from build123d import *

# Parameters (mm, degrees)
F0_R         = 7.62
F1_DEPTH     = 19.05
F3_DEPTH     = 12.7
F4_SIZE      = 1.27
F5_T1_DEPTH  = 8.5497045256
F5_T3_DEPTH  = 8.5497045256
F5_T5_DEPTH  = 8.5497045256
F5_T7_DEPTH  = 8.5497045256
F5_T12_DEPTH = 8.5497045256
F5_S13_R     = 7.62
F5_T14_DEPTH = 6
F5_T18_DEPTH = 8.5497045256
F5_S19_R     = 7.62
F5_T20_DEPTH = 6
F5_T24_DEPTH = 8.5497045256
F5_S25_R     = 7.62
F5_T26_DEPTH = 6
F5_T30_DEPTH = 8.5497045256
F5_S31_R     = 7.62
F5_T32_DEPTH = 6
F5_T36_DEPTH = 8.5497045256
F5_S37_R     = 7.62
F5_T38_DEPTH = 6
F5_T42_DEPTH = 8.5497045256
F5_S43_R     = 7.62
F5_T44_DEPTH = 6
F6_R         = 7.62
F7_DEPTH     = 12.7
F8_R         = 6.35
F9_DEPTH     = 44.4510001


# Not quite as in the source:
# - a fillet or chamfer that OpenCascade refuses, or shapes differently, is made with other operations: its cross-section is extruded or revolved along the edge and cut away or added


with BuildPart() as f1:
    # F0 (on Front) → F1 (new body)
    with BuildSketch(Plane.XZ):
        Circle(F0_R)
    extrude(amount=F1_DEPTH)

    # F2 (on face) → F3 (join)
    with BuildSketch(Plane.XZ.offset(19.05)):
        with BuildLine():
            Line((7.8629215405, 3.9488814679), (4.1872753391, 6.3664059904))
            ThreePointArc((4.1872753391, 6.3664059904), (6.7071394083, 3.6164459015), (7.62, 0))
            ThreePointArc((7.62, 0), (7.616776064, -0.2216357159), (7.6071069841, -0.4430838887))
            Line((7.6071069841, -0.4430838887), (7.8629215405, 3.9488814679))
        make_face()
        with BuildLine():
            ThreePointArc((4.1872753391, 6.3664059904), (0.4430838236, 7.6071069879), (-3.4198316443, 6.8094898138))
            ThreePointArc((-3.4198316443, 6.8094898138), (-6.3664059346, 4.187275424), (-7.6071069765, 0.4430840189))
            ThreePointArc((-7.6071069765, 0.4430840189), (-6.8094898664, -3.4198315396), (-4.187275378, -6.3664059648))
            ThreePointArc((-4.187275378, -6.3664059648), (-0.4430838337, -7.6071069873), (3.419831668, -6.8094898019))
            ThreePointArc((3.419831668, -6.8094898019), (6.3664059777, -4.1872753585), (7.6071069841, -0.4430838887))
            ThreePointArc((7.6071069841, -0.4430838887), (7.616776064, -0.2216357159), (7.62, 0))
            ThreePointArc((7.62, 0), (6.7071394083, 3.6164459015), (4.1872753391, 6.3664059904))
        make_face()
        with BuildLine():
            ThreePointArc((7.6071069841, -0.4430838887), (6.3664059777, -4.1872753585), (3.419831668, -6.8094898019))
            Line((3.419831668, -6.8094898019), (7.351292438, -4.8350490681))
            Line((7.351292438, -4.8350490681), (7.6071069841, -0.4430838887))
        make_face()
        with BuildLine():
            ThreePointArc((3.419831668, -6.8094898019), (-0.4430838337, -7.6071069873), (-4.187275378, -6.3664059648))
            Line((-4.187275378, -6.3664059648), (-0.5116291025, -8.783930536))
            Line((-0.5116291025, -8.783930536), (3.419831668, -6.8094898019))
        make_face()
        with BuildLine():
            ThreePointArc((-4.187275378, -6.3664059648), (-6.8094898664, -3.4198315396), (-7.6071069765, 0.4430840189))
            Line((-7.6071069765, 0.4430840189), (-7.8629215405, -3.9488814679))
            Line((-7.8629215405, -3.9488814679), (-4.187275378, -6.3664059648))
        make_face()
        with BuildLine():
            Line((-3.4198316443, 6.8094898138), (-7.351292438, 4.8350490681))
            Line((-7.351292438, 4.8350490681), (-7.6071069765, 0.4430840189))
            ThreePointArc((-7.6071069765, 0.4430840189), (-6.3664059346, 4.187275424), (-3.4198316443, 6.8094898138))
        make_face()
        with BuildLine():
            Line((0.5116291025, 8.783930536), (-3.4198316443, 6.8094898138))
            ThreePointArc((-3.4198316443, 6.8094898138), (0.4430838236, 7.6071069879), (4.1872753391, 6.3664059904))
            Line((4.1872753391, 6.3664059904), (0.5116291025, 8.783930536))
        make_face()
    extrude(amount=F3_DEPTH)

    # F4
    f4_edges = [f1.edges().sort_by_distance(p)[0] for p in [
        (7.862922, -25.4, 3.948881),
        (7.351292, -25.4, -4.835049),
        (-0.511629, -25.4, -8.783931),
        (-7.862922, -25.4, -3.948881),
        (-7.351292, -25.4, 4.835049),
        (0.511629, -25.4, 8.783931),
    ]]
    chamfer(f4_edges, length=F4_SIZE)

    # F5: fillet of radius 1.27 on 12 edges, made by hand

    # F5_s2 → F5_t1 (cut)
    with BuildSketch(Plane(origin=(1.918540045, 0, -3.8201526101), x_dir=(0, 1, 0), z_dir=(-0.4487968068, 0, 0.8936338323))):
        with BuildLine():
            ThreePointArc((-30.48, -8.1638181024), (-31.3780256121, -7.7918437146), (-31.75, -6.8938181024))
            Line((-31.75, -6.8938181024), (-31.75, -8.1638181024))
            Line((-31.75, -8.1638181024), (-30.48, -8.1638181024))
        make_face()
        with BuildLine():
            ThreePointArc((-31.75, 6.8938181024), (-31.3780256121, 7.7918437146), (-30.48, 8.1638181024))
            Line((-30.48, 8.1638181024), (-31.75, 8.1638181024))
            Line((-31.75, 8.1638181024), (-31.75, 6.8938181024))
        make_face()
    extrude(amount=F5_T1_DEPTH, mode=Mode.SUBTRACT)

    # F5_s4 → F5_t3 (cut)
    with BuildSketch(Plane(origin=(4.2676192292, 0, -0.2485718879), x_dir=(0, 1, 0), z_dir=(-0.9983080038, 0, 0.0581474803))):
        with BuildLine():
            ThreePointArc((-31.75, -6.8938181024), (-31.3780256121, -7.7918437146), (-30.48, -8.1638181024))
            Line((-30.48, -8.1638181024), (-31.75, -8.1638181024))
            Line((-31.75, -8.1638181024), (-31.75, -6.8938181024))
        make_face()
        with BuildLine():
            ThreePointArc((-31.75, 6.8938181024), (-31.3780256121, 7.7918437146), (-30.48, 8.1638181024))
            Line((-30.48, 8.1638181024), (-31.75, 8.1638181024))
            Line((-31.75, 8.1638181024), (-31.75, 6.8938181024))
        make_face()
    extrude(amount=F5_T3_DEPTH, mode=Mode.SUBTRACT)

    # F5_s6 → F5_t5 (cut)
    with BuildSketch(Plane(origin=(-2.3490791841, 0, -3.5715807222), x_dir=(0, 1, 0), z_dir=(0.5495111971, 0, 0.835486352))):
        with BuildLine():
            ThreePointArc((-31.75, 6.8938181024), (-31.3780256121, 7.7918437146), (-30.48, 8.1638181024))
            Line((-30.48, 8.1638181024), (-31.75, 8.1638181024))
            Line((-31.75, 8.1638181024), (-31.75, 6.8938181024))
        make_face()
    extrude(amount=F5_T5_DEPTH, mode=Mode.SUBTRACT)

    # F5_s8 → F5_t7 (cut)
    with BuildSketch(Plane(origin=(2.3490791841, 0, 3.5715807222), x_dir=(0, 1, 0), z_dir=(-0.5495111971, 0, -0.835486352))):
        with BuildLine():
            ThreePointArc((-30.48, 8.1638181024), (-31.3780256121, 7.7918437146), (-31.75, 6.8938181024))
            Line((-31.75, 6.8938181024), (-31.75, 8.1638181024))
            Line((-31.75, 8.1638181024), (-30.48, 8.1638181024))
        make_face()
    extrude(amount=F5_T7_DEPTH, mode=Mode.SUBTRACT)


with BuildPart() as f5_tool10:
    # F5_s11 → F5_t12 (new body)
    with BuildSketch(Plane(origin=(4.2676192292, 0, -0.2485718879), x_dir=(0, 1, 0), z_dir=(-0.9983080038, 0, 0.0581474803))):
        with BuildLine():
            ThreePointArc((-19.05, -6.8938181024), (-19.4219743879, -7.7918437146), (-20.32, -8.1638181024))
            Line((-20.32, -8.1638181024), (-19.05, -8.1638181024))
            Line((-19.05, -8.1638181024), (-19.05, -6.8938181024))
        make_face()
    extrude(amount=F5_T12_DEPTH)

    # F5_s13 → F5_t14 (cut, symmetric)
    with BuildSketch(Plane.XZ.offset(19.7)):
        Circle(F5_S13_R)
    extrude(amount=F5_T14_DEPTH, both=True, mode=Mode.SUBTRACT)


with BuildPart() as f1_1:
    add(f1.part)

    # F5_t9: cut F5_tool10
    add(f5_tool10.part, mode=Mode.SUBTRACT)


with BuildPart() as f5_tool16:
    # F5_s17 → F5_t18 (new body)
    with BuildSketch(Plane(origin=(-2.3490791841, 0, -3.5715807222), x_dir=(0, 1, 0), z_dir=(0.5495111971, 0, 0.835486352))):
        with BuildLine():
            ThreePointArc((-19.05, 6.8938181024), (-19.4219743879, 7.7918437146), (-20.32, 8.1638181024))
            Line((-20.32, 8.1638181024), (-19.05, 8.1638181024))
            Line((-19.05, 8.1638181024), (-19.05, 6.8938181024))
        make_face()
    extrude(amount=F5_T18_DEPTH)

    # F5_s19 → F5_t20 (cut, symmetric)
    with BuildSketch(Plane.XZ.offset(19.7)):
        Circle(F5_S19_R)
    extrude(amount=F5_T20_DEPTH, both=True, mode=Mode.SUBTRACT)


with BuildPart() as f1_2:
    add(f1_1.part)

    # F5_t15: cut F5_tool16
    add(f5_tool16.part, mode=Mode.SUBTRACT)


with BuildPart() as f5_tool22:
    # F5_s23 → F5_t24 (new body)
    with BuildSketch(Plane(origin=(1.918540045, 0, -3.8201526101), x_dir=(0, 1, 0), z_dir=(-0.4487968068, 0, 0.8936338323))):
        with BuildLine():
            ThreePointArc((-19.05, 6.8938181024), (-19.4219743879, 7.7918437146), (-20.32, 8.1638181024))
            Line((-20.32, 8.1638181024), (-19.05, 8.1638181024))
            Line((-19.05, 8.1638181024), (-19.05, 6.8938181024))
        make_face()
    extrude(amount=F5_T24_DEPTH)

    # F5_s25 → F5_t26 (cut, symmetric)
    with BuildSketch(Plane.XZ.offset(19.7)):
        Circle(F5_S25_R)
    extrude(amount=F5_T26_DEPTH, both=True, mode=Mode.SUBTRACT)


with BuildPart() as f1_3:
    add(f1_2.part)

    # F5_t21: cut F5_tool22
    add(f5_tool22.part, mode=Mode.SUBTRACT)


with BuildPart() as f5_tool28:
    # F5_s29 → F5_t30 (new body)
    with BuildSketch(Plane(origin=(4.2676192292, 0, -0.2485718879), x_dir=(0, 1, 0), z_dir=(-0.9983080038, 0, 0.0581474803))):
        with BuildLine():
            ThreePointArc((-19.05, 6.8938181024), (-19.4219743879, 7.7918437146), (-20.32, 8.1638181024))
            Line((-20.32, 8.1638181024), (-19.05, 8.1638181024))
            Line((-19.05, 8.1638181024), (-19.05, 6.8938181024))
        make_face()
    extrude(amount=F5_T30_DEPTH)

    # F5_s31 → F5_t32 (cut, symmetric)
    with BuildSketch(Plane.XZ.offset(19.7)):
        Circle(F5_S31_R)
    extrude(amount=F5_T32_DEPTH, both=True, mode=Mode.SUBTRACT)


with BuildPart() as f1_4:
    add(f1_3.part)

    # F5_t27: cut F5_tool28
    add(f5_tool28.part, mode=Mode.SUBTRACT)


with BuildPart() as f5_tool34:
    # F5_s35 → F5_t36 (new body)
    with BuildSketch(Plane(origin=(2.3490791841, 0, 3.5715807222), x_dir=(0, 1, 0), z_dir=(-0.5495111971, 0, -0.835486352))):
        with BuildLine():
            ThreePointArc((-19.05, 6.8938181024), (-19.4219743879, 7.7918437146), (-20.32, 8.1638181024))
            Line((-20.32, 8.1638181024), (-19.05, 8.1638181024))
            Line((-19.05, 8.1638181024), (-19.05, 6.8938181024))
        make_face()
    extrude(amount=F5_T36_DEPTH)

    # F5_s37 → F5_t38 (cut, symmetric)
    with BuildSketch(Plane.XZ.offset(19.7)):
        Circle(F5_S37_R)
    extrude(amount=F5_T38_DEPTH, both=True, mode=Mode.SUBTRACT)


with BuildPart() as f1_5:
    add(f1_4.part)

    # F5_t33: cut F5_tool34
    add(f5_tool34.part, mode=Mode.SUBTRACT)


with BuildPart() as f5_tool40:
    # F5_s41 → F5_t42 (new body)
    with BuildSketch(Plane(origin=(1.918540045, 0, -3.8201526101), x_dir=(0, 1, 0), z_dir=(-0.4487968068, 0, 0.8936338323))):
        with BuildLine():
            ThreePointArc((-19.05, -6.8938181024), (-19.4219743879, -7.7918437146), (-20.32, -8.1638181024))
            Line((-20.32, -8.1638181024), (-19.05, -8.1638181024))
            Line((-19.05, -8.1638181024), (-19.05, -6.8938181024))
        make_face()
    extrude(amount=F5_T42_DEPTH)

    # F5_s43 → F5_t44 (cut, symmetric)
    with BuildSketch(Plane.XZ.offset(19.7)):
        Circle(F5_S43_R)
    extrude(amount=F5_T44_DEPTH, both=True, mode=Mode.SUBTRACT)


with BuildPart() as f1_6:
    add(f1_5.part)

    # F5_t39: cut F5_tool40
    add(f5_tool40.part, mode=Mode.SUBTRACT)

    # F6 (on face) → F7 (join)
    with BuildSketch(Plane.XZ.offset(31.75)):
        Circle(F6_R)
    extrude(amount=F7_DEPTH)

    # F8 (on face) → F9 (cut, through all)
    with BuildSketch(Plane.XZ.offset(44.45)):
        Circle(F8_R)
    extrude(amount=-F9_DEPTH, mode=Mode.SUBTRACT)


solid = f1_6.part
Geometry: final body of the model. Coordinates: model frame, mm. A direction names the side the tool comes from. Round coordinates to 2 decimals unless told otherwise and drop trailing zeros. Loops run counter-clockwise (first coordinate to the right, second up) from the corner with the lowest first, then second, coordinate; pieces in that order, holes last. Notation, with made-up numbers: M -33,89.25 L -29,89.25 A18 cw -29,96.25 Z; hole C 52,-33 d8. An arc over 180 degrees is marked long. Put each result on its own line as item: value. Start each with the question number.
(1) Draft query along X for faces 4 (the face through (-6.8, -31.5, -3.5)), 5 (the face through (0.46, -25.33, 8.15)), 6 (the face through (-1.65, -38.01, -7.44)). Return one class per face: +X half, -X half, draft (parallel to the pull), parting line (faces both ways), or undercut.
(2) Material intervals for line 1 along Z through (x, y) = (0, -17); line 2 along X through (y, z) = (-1.5, 5), sorted ascending. Write a range as [from, to].
(3) Section query B-B (y = -14). Return loops of the section in (x, z).
(4) Section query A-A (y = -21). Return loops of the section in (x, z), then the cut area to 3 significant figures.
(5) Set-up query: faces 1 (the face through (7.302, -25.329, 3.65)), 2 (the face through (-1.65, -9.5, -7.44)), 3 (the face through (-6.38, -31.53, 4.14)). Return all of +Z, -Z, +X, -X, +Y, -Y with unobstructed straight access to the full face (end or side cutting, diameter ignored); none if empty.
(6) Contact query for flat-ended pins moving along their axis: pin 1 Ø3 at (y, z) = (-13.5, -5) entering from +X; pin 2 Ø5 at (y, z) = (-25.5, 1) entering from -X; pin 3 Ø1 at (y, z) = (-13.5, -6.5) entering from +X. Output: stop coordinate, or through.
Findings below:
1. face 4: undercut
1. face 5: +X half
1. face 6: parting line
2. line 1: z = [-7.62, -6.35], [6.35, 7.62]
2. line 2: x = [-5.75, -3.91], [3.91, 5.75]
3. outline: C 0,0 d15.24; hole C 0,0 d12.7
4. outline: M -7.79,-2.68 L -6.8,-4.65 L -1.57,-8.09 L 0.62,-8.21 L 6.22,-5.41 L 7.43,-3.57 L 7.79,2.68 L 6.8,4.65 L 1.57,8.09 L -0.62,8.21 L -6.22,5.41 L -7.43,3.57 Z; hole C 0,0 d12.7
4. area: 70.3 mm2
5. face 1: +Z, +X, +Y, -Y
5. face 2: +Y
5. face 3: none
6. pin 1: stops at x = 6.77
6. pin 2: stops at x = -7.72
6. pin 3: stops at x = 4.7
